Read the model definition and answer for the solid it produces. Units are mm, in the model's axes. Face numbers are marked on the shaded views. A direction names the side the tool comes from. Coordinates: 2 decimals unless noted, no trailing zeros. Write each loop counter-clockwise with the first axis right and the second up, starting at its lowest first coordinate (ties: lowest second). Pieces come first, ordered by that corner, then holes. Notation, with made-up numbers: (14, -4.5) -> (70, -4.5) arc R21 ccw to (70, 11.5) -> close; hole circle Ø4 at (22.25, 47). An arc over 180 degrees is marked (long way). One line per item, written item: value. Start each with the question number.
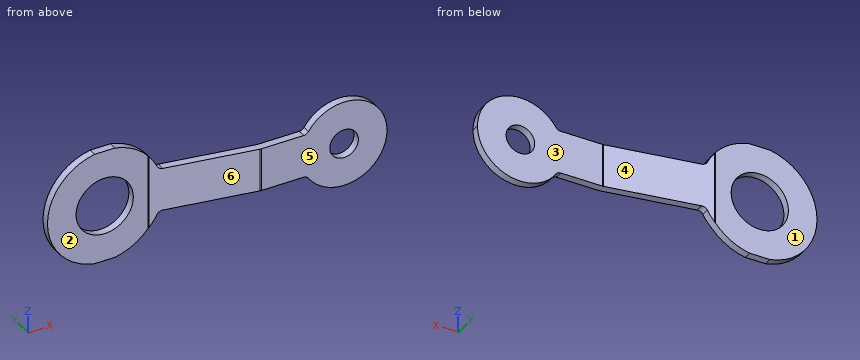
from build123d import *

# Parameters (mm, degrees)
F0_R     = 25.4
F0_R_2   = 12.7
F1_DEPTH = 25.4
F3_DEPTH = 50
F4_R     = 5.08


with BuildPart() as f1:
    # F0 (on Front) → F1 (new body)
    with BuildSketch(Plane.XZ):
        with BuildLine():
            ThreePointArc((47.09286, -19.05), (49.864603, -9.703677), (50.8, 0))
            ThreePointArc((50.8, 0), (49.864603, 9.703677), (47.09286, 19.05))
            ThreePointArc((47.09286, 19.05), (-50.8, 0), (47.09286, -19.05))
        make_face()
        Circle(F0_R, mode=Mode.SUBTRACT)
        with BuildLine():
            ThreePointArc((47.09286, 19.05), (49.864603, 9.703677), (50.8, 0))
            ThreePointArc((50.8, 0), (49.864603, -9.703677), (47.09286, -19.05))
            Line((47.09286, -19.05), (170.204432, -19.05))
            ThreePointArc((170.204432, -19.05), (165.1, 0), (170.204432, 19.05))
            Line((170.204432, 19.05), (47.09286, 19.05))
        make_face()
        with BuildLine():
            ThreePointArc((241.3, 0), (213.061006, 36.801774), (170.204432, 19.05))
            ThreePointArc((170.204432, 19.05), (165.1, 0), (170.204432, -19.05))
            ThreePointArc((170.204432, -19.05), (213.061006, -36.801774), (241.3, 0))
        make_face()
        with Locations((203.2, 0)):
            Circle(F0_R_2, mode=Mode.SUBTRACT)
    extrude(amount=F1_DEPTH)

    # F2 (on Top) → F3 (intersect, symmetric)
    with BuildSketch(Plane.XY):
        Polygon((39.602962, 0), (-68.855375, 0), (-68.855375, -6.858), (39.002964, -6.858), (129.294157, -22.778774), (255.28869, -22.778774), (255.28869, -15.920773), (129.894154, -15.920773), align=None)
    extrude(amount=F3_DEPTH, both=True, mode=Mode.INTERSECT)

    # F4
    f4_edges = [f1.edges().sort_by_distance(p)[0] for p in [
        (129.894154, -15.920773, 0),
        (39.602962, 0, 0),
        (39.002964, -6.858, 0),
        (129.294157, -22.778774, 0),
        (47.09286, -4.802569, 19.05),
        (170.204432, -19.349774, 19.05),
        (170.204432, -19.349774, -19.05),
        (47.09286, -4.802569, -19.05),
    ]]
    fillet(f4_edges, radius=F4_R)


solid = f1.part
1. A tool of negligible diameter and unlimited length cuts with its end or side. For the marked faces 1, 2 and 3, from which of +Z, -Z, +X, -X, +Y, -Y can it reach the whole face along a straight path? Write none if from no direction.
2. A cutting plane is placed at B-B on x = 209. Give the vertices of the cut face in (y, z), then the cut area to 3 significant figures.
3. For a pull along X with two mould halves and no side action, classify the marked faces 4, 5 and 6 as +X half, -X half, draft (parallel to the pull), parting line (faces both ways), or undercut.
4. A cutting plane is placed at A-A on x = 0. Give the vertices of the cut face in (y, z), then the cut area to 3 significant figures.
5. Find the intervals of material crossed by probe 1 along Z at (x, y) = (203.2, -17.75); probe 2 along Z at (x, y) = (0, -4.25); probe 3 along Y at (x, z) = (182, -2.5), in increasing order. Write a range as from..to.
6. Given pin 1 (12 mm diameter, centred on x = 96, z = -23.5, fed in from -Y); pin 2 (3 mm diameter, centred on x = 34.5, y = -4, fed in from -Z); pin 3 (4 mm diameter, centred on y = -6, z = -31.5, fed in from +X), each flat-ended and moving along its own axis, determine where each tip first touches the part or whether it passes through.
7. A cutting plane is placed at C-C on x = 53. Give the vertices of the cut face in (y, z), then the cut area to 3 significant figures.
Derived:
1. face 1: +Z, -Z, +X, -X, +Y
1. face 2: +Z, -Z, -X, -Y
1. face 3: +Z, -Z, +X, +Y
2. outline: (-22.78, -37.66) -> (-15.92, -37.66) -> (-15.92, -11.3) -> (-22.78, -11.3) -> close; (-22.78, 11.3) -> (-15.92, 11.3) -> (-15.92, 37.66) -> (-22.78, 37.66) -> close
2. area: 362 mm2
3. face 4: +X half
3. face 5: draft
3. face 6: -X half
4. outline: (-6.86, -50) -> (0, -50) -> (0, -25.4) -> (-6.86, -25.4) -> close; (-6.86, 25.4) -> (0, 25.4) -> (0, 50) -> (-6.86, 50) -> close
4. area: 337 mm2
5. probe 1: z = -38.1..-12.7, 12.7..38.1
5. probe 2: z = -50..-25.4, 25.4..50
5. probe 3: y = -22.78..-15.92
6. pin 1: stops at y = -17.62
6. pin 2: stops at z = -38.62
6. pin 3: stops at x = 41.36
7. outline: (-9.33, -19.05) -> (-2.36, -19.05) -> (-2.36, 19.05) -> (-9.33, 19.05) -> close
7. area: 265 mm2
